For this review, take the finished solid that the model builds, in its own axes (mm). Face numbers are marked on the shaded views. Give positions to 0.01 mm unless a question says otherwise; leave off trailing zeros. Order: outer loops, then holes, each group sorted by start corner. A loop starts at its lowest first (then second) coordinate and runs counter-clockwise, first axis right, second up. Notation, with made-up numbers: M -19.5,62.5 L 27.5,62.5 A22 ccw 27.5,71.5 Z; hole C 61,81 d4. An arc over 180 degrees is marked long. Use CSV: the item, a comma, the result in double quotes. Start each with the question number.
(1) Consider section D-D (y = 8.75). Write out the cut boundary in (x, z), and give its area (3 significant figures).
(2) Consider section B-B (z = 18.5). Write out the cut boundary in (x, y).
(3) Clearance check with flat-ended pins moving along their axes: P1, Ø13, axis at x = -15.33, z = 38.89, coming from the -Y side; P2, Ø12, axis at x = 0, z = 24.38, coming from the +Y side. State where each tip first meets the part, or that it passes through.
(4) Consider section A-A (x = -6). Write out the cut boundary in (y, z).
(5) Consider section C-C (z = -41). Write out the cut boundary in (x, y).
(6) Wall thickness on L1, parallel to Z at x = 0, y = 6; L2, parallel to Z at x = 16, y = 9; L3, parallel to X at y = -3.5, z = -38: over which ranges is each line inside the solid? List them lowest first. Write a range as from..to.
(7) Draft analysis for pull direction Z (two halves, no side actions). For the marked faces 1, 2 and 3, state which applies: pulls with the +Z half, pulls with the -Z half, needs draft (parallel to the pull), parting line crosses it, or undercut.
```python
from build123d import *

# Parameters (mm, degrees)
F0_W     = 50.8
F0_H     = 101.6
F0_R     = 7.62
F1_DEPTH = 12.7
F2_R     = 5.08
F3_R     = 5.092996
F4_DEPTH = 25.4


with BuildPart() as f1:
    # F0 (on Front) → F1 (new body, symmetric)
    with BuildSketch(Plane.XZ):
        Rectangle(F0_W, F0_H)
        with Locations((0, -24.378773)):
            Circle(F0_R, mode=Mode.SUBTRACT)
        with Locations((0, 24.378773)):
            Circle(F0_R, mode=Mode.SUBTRACT)
    extrude(amount=F1_DEPTH, both=True)

    # F2
    f2_edges = [f1.edges().sort_by_distance(p)[0] for p in [
        (25.4, 0, 50.8),
        (-25.4, 0, 50.8),
        (25.4, 0, -50.8),
        (-25.4, 0, -50.8),
    ]]
    fillet(f2_edges, radius=F2_R)

    # F3 (on face) → F4 (cut, through all)
    with BuildSketch(Plane.XZ.offset(12.7)):
        with Locations((-15.331865, 38.888112)):
            Circle(F3_R)
        with Locations((15.331865, 38.888112)):
            Circle(F3_R)
        with Locations((15.331865, -38.888112)):
            Circle(F3_R)
        with Locations((-15.331865, -38.888112)):
            Circle(F3_R)
    extrude(amount=-F4_DEPTH, mode=Mode.SUBTRACT)


solid = f1.part
```
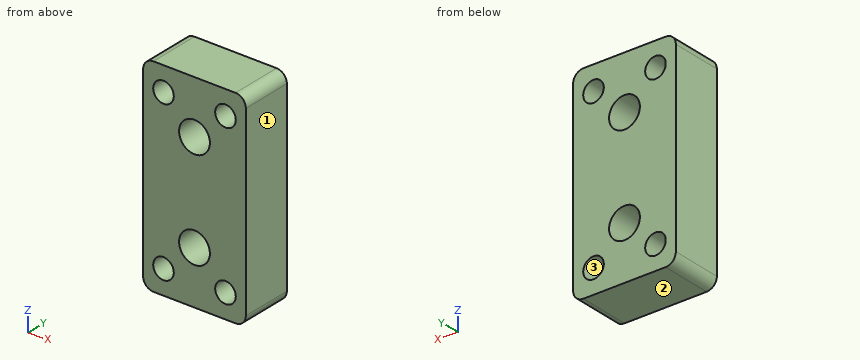
Check result:
1,outline,"M -25.4,-45.72 A5.08 ccw -20.32,-50.8 L 20.32,-50.8 A5.08 ccw 25.4,-45.72 L 25.4,45.72 A5.08 ccw 20.32,50.8 L -20.32,50.8 A5.08 ccw -25.4,45.72 Z; hole C -15.33,-38.89 d10.19; hole C -15.33,38.89 d10.19; hole C 0,-24.38 d15.24; hole C 0,24.38 d15.24; hole C 15.33,-38.89 d10.19; hole C 15.33,38.89 d10.19"
1,area,"4,450 mm^2"
2,outline,"M -25.4,-12.7 L -4.85,-12.7 L -4.85,12.7 L -25.4,12.7 Z; M 4.85,-12.7 L 25.4,-12.7 L 25.4,12.7 L 4.85,12.7 Z"
3,P1,"stops at y = -12.7"
3,P2,"passes through"
4,outline,"M -12.7,-50.8 L 12.7,-50.8 L 12.7,-29.08 L -12.7,-29.08 Z; M -12.7,-19.68 L 12.7,-19.68 L 12.7,19.68 L -12.7,19.68 Z; M -12.7,29.08 L 12.7,29.08 L 12.7,50.8 L -12.7,50.8 Z"
5,outline,"M -25.4,-12.7 L -19.97,-12.7 L -19.97,12.7 L -25.4,12.7 Z; M -10.7,-12.7 L 10.7,-12.7 L 10.7,12.7 L -10.7,12.7 Z; M 19.97,-12.7 L 25.4,-12.7 L 25.4,12.7 L 19.97,12.7 Z"
6,L1,"z = -50.8..-32, -16.76..16.76, 32..50.8"
6,L2,"z = -50.8..-43.94, -33.84..33.84, 43.94..50.8"
6,L3,"x = -25.4..-20.35, -10.32..10.32, 20.35..25.4"
7,face 1,"needs draft"
7,face 2,"pulls with the -Z half"
7,face 3,"undercut"
